Model file for the job. Use its own axes, mm. A direction names the side the tool comes from. Coordinates: 2 decimals unless noted, no trailing zeros. Loops run counter-clockwise (first coordinate to the right, second up) from the corner with the lowest first, then second, coordinate; pieces in that order, holes last. Notation, with made-up numbers: M 54.5,14 L 82.5,14 A25 cw 82.5,44 Z; hole C 40.25,52.5 d3. An arc over 180 degrees is marked long. Write item = value, one per line. Start each with the question number.
Autodesk Inventor part; units mm, degrees
ref_plane "Work Plane1" through (13.25, 0, 31.1) normal (1, 0, 0) x (0, 1, 0)
ref_plane "YZ Plane" through (0, 0, 0) normal (1, 0, 0) x (0, 1, 0)
ref_plane "XZ Plane" through (0, 0, 0) normal (0, 1, 0) x (-1, 0, 0)
sketch "Sketch1" plane through (0, 0, 0) normal (0, 0, 1) x (1, 0, 0)
  circle A0 centre (0, 0) radius 25
  dimension "d0" = 50
extrude "Extrusion1" add sketch "Sketch1" along normal blind 16
sketch "Sketch2" plane through (0, 0, 16) normal (0, 0, 1) x (1, 0, 0)
  line L0 (0, 0) -> (-14.1421, 14.1421)
  line L1 (0, 0) -> (-17.9491, 0)
  point P0 (-14.1421, -14.1421)
  point P1 (-14.1421, -14.1421)
  point P2 (14.1421, -14.1421)
  point P3 (14.1421, -14.1421)
  point P4 (14.1421, 14.1421)
  point P5 (14.1421, 14.1421)
  point P6 (0, 20)
  dimension "d3" = 45
  dimension "d4" = 20
  dimension "d7" = 360
  dimension "d9" = 20
hole "Hole1" at (-14.1421, 14.1421, 16) at (-14.1421, -14.1421, 16) at (14.1421, -14.1421, 16) at (14.1421, 14.1421, 16) at (0, 20, 16) direction (0, 0, -1) diameter 6.5 end through all
sketch "Sketch3" plane through (0, 0, 16) normal (0, 0, 1) x (1, 0, 0)
  circle A0 centre (0, 0) radius 13.25
  dimension "d17" = 26.5
extrude "Extrusion2" add sketch "Sketch3" along normal blind 15.1
sketch "Sketch4" plane through (0, 0, 31.1) normal (0, 0, 1) x (1, 0, 0)
  circle A0 centre (0, 0) radius 13.25
  point P0 (13.25, 0)
ref_plane "Work Plane1" through (13.25, 0, 31.1) normal (1, 0, 0) x (0, 1, 0)
properties part number "SoporteIRB"
Item 1: Pull direction Y, two halves, no side cores. Call faces 1 (the cylindrical face through (23.846, -7.509, 7.888)), 2 (the cylindrical face through (-0.143, 23.247, 7.888)), 3 (the flat face through (0, 0, 31.1)): +Y half, -Y half, draft (parallel to the pull), parting line (faces both ways), or undercut.
Item 2: Cut at B-B (y = 20). Give the cut face in (x, z).
Item 3: Cut at A-A (x = 0). Give the cut face in (y, z), plus the area to 3 significant figures.
Item 4: 3-axis set-ups, long thin cutter, end or side, ignore diameter. For faces 4 (the flat face through (11, -11, 16)), 5 (the cylindrical face through (-17.364, 14.565, 7.888)): which of +Z, -Z, +X, -X, +Y, -Y reach the whole face in a straight line?
Item 5: Cut at C-C (y = 0). Give the cut face in (x, z), plus the area to 3 significant figures.
Item 6: Cut at D-D (y = -15.5). Give the cut face in (x, z), plus the area to 3 significant figures.
Item 7: Pin check, flat tips, straight feed: pin 1 Ø5 at (x, z) = (8.5, 15.5) entering from -Y; pin 2 Ø5 at (y, z) = (11.5, 20.5) entering from +X; pin 3 Ø6 at (x, z) = (9.5, 20.5) entering from -Y. Stop position of each tip, or through.
Item 8: Probe L1, parallel to Y at x = 13.5, z = 15.5; L2, parallel to Y at x = 15.5, z = 8.5; L3, parallel to Z at x = 20, y = -1. List the from-to ranges inside material, lowest first.
Reported:
q1.face_1 = parting line
q1.face_2 = undercut
q1.face_3 = draft
q2.outline = M -15,0 L -3.25,0 L -3.25,16 L -15,16 Z; M 3.25,0 L 15,0 L 15,16 L 3.25,16 Z
q3.outline = M -25,0 L 16.75,0 L 16.75,16 L 13.25,16 L 13.25,31.1 L -13.25,31.1 L -13.25,16 L -25,16 Z; M 23.25,0 L 25,0 L 25,16 L 23.25,16 Z
q3.area = 1,100 mm^2
q4.face_4 = +Z
q4.face_5 = +Z, -Z
q5.outline = M -25,0 L 25,0 L 25,16 L 13.25,16 L 13.25,31.1 L -13.25,31.1 L -13.25,16 L -25,16 Z
q5.area = 1,200 mm^2
q6.outline = M -19.62,0 L -17.09,0 L -17.09,16 L -19.62,16 Z; M -11.19,0 L 11.19,0 L 11.19,16 L -11.19,16 Z; M 17.09,0 L 19.62,0 L 19.62,16 L 17.09,16 Z
q6.area = 439 mm^2
q7.pin_1 = -24.27
q7.pin_2 = 9.72
q7.pin_3 = -11.55
q8.L1 = -21.04 to -17.33, -10.96 to 10.96, 17.33 to 21.04
q8.L2 = -19.62 to -17.09, -11.19 to 11.19, 17.09 to 19.62
q8.L3 = 0 to 16
